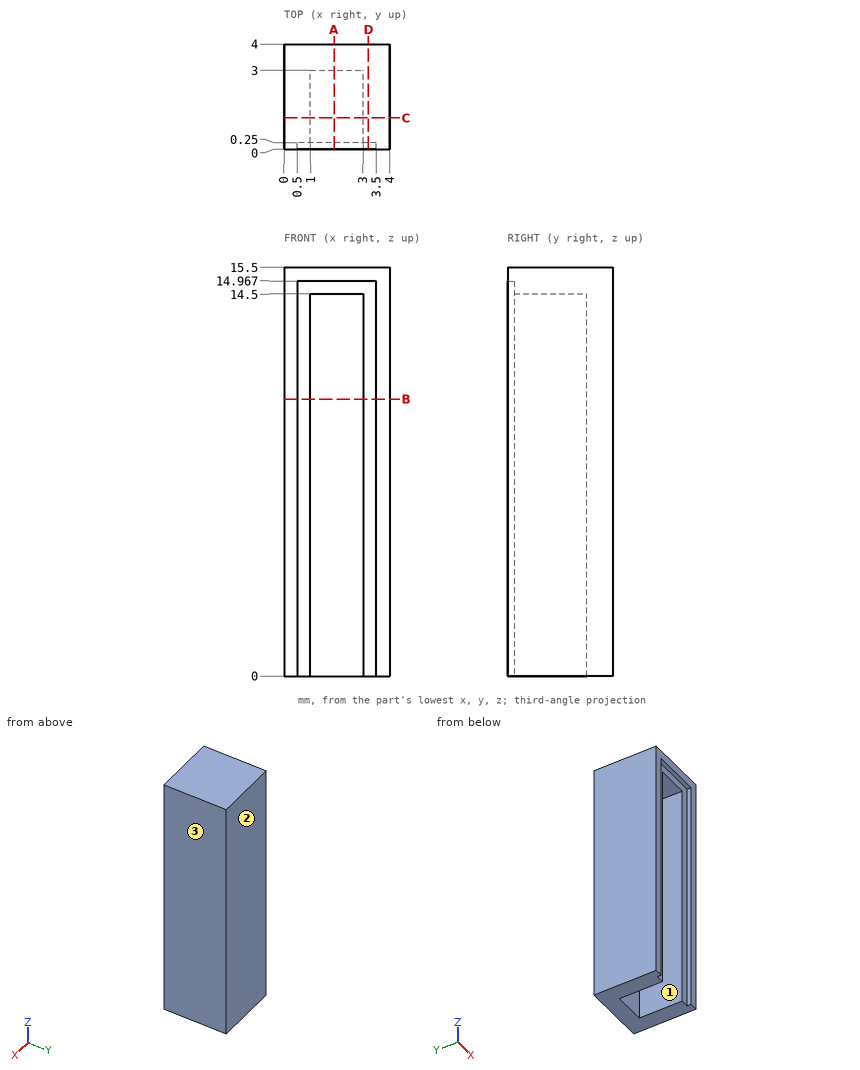
Could you check a few things on this drawing? It's one solid part, dimensions in mm from its lowest x, y, z. Round coordinates to 2 decimals unless told otherwise and drop trailing zeros. Order: outer loops, then holes, each group sorted by start corner. A loop starts at its lowest first (then second) coordinate and runs counter-clockwise, first axis right, second up. Notation, with made-up numbers: (-34.5, 40) -> (19.5, 40) arc R34 ccw to (19.5, 70) -> close; hole circle Ø1 at (76.25, -22.75). An arc over 180 degrees is marked (long way). One line per question, with ' | ' between items.
Q1. We'd pull the mould along X, two halves only. Please class the marked faces 1, 2 and 3: released by +X, released by -X, zero draft, split by the parting line, or undercut.
Computed values:
face 1: undercut | face 2: zero draft | face 3: released by +X
Q2. If I drill on line 1 (X direction, y = 1.9, z = 10.25); line 2 (Y direction, x = 1.65, z = 7); line 3 (Z direction, x = 1.9, y = 2.3), over which ranges is the centre line in solid material (lowest first)? Write a range as from..to.
Computed values:
line 1: 0..1, 3..4 | line 2: 3..4 | line 3: 14.5..15.5
Q3. I'm going to push flat-ended pins straight in: pin 1 (0.6 mm diameter, centred on x = 1.5, z = 9, fed in from -Y); pin 2 (1.5 mm diameter, centred on x = 2.5, z = 11, fed in from -Y). Where does each tip first touch, or does it pass through?
Computed values:
pin 1: y = 3 | pin 2: y = 0.25
Q4. If we section it at D-D on x = 3.2: Write out the boundary of the cut face in (y, z).
Computed values:
outline: (0, 14.97) -> (0.25, 14.97) -> (0.25, 0) -> (4, 0) -> (4, 15.5) -> (0, 15.5) -> close
Q5. If we section it at B-B on z = 10.5: Write out the boundary of the cut face in (x, y).
Computed values:
outline: (0, 0) -> (0.5, 0) -> (0.5, 0.25) -> (1, 0.25) -> (1, 3) -> (3, 3) -> (3, 0.25) -> (3.5, 0.25) -> (3.5, 0) -> (4, 0) -> (4, 4) -> (0, 4) -> close
Q6. If we section it at C-C on y = 1.2: Write out the boundary of the cut face in (x, z).
Computed values:
outline: (0, 0) -> (1, 0) -> (1, 14.5) -> (3, 14.5) -> (3, 0) -> (4, 0) -> (4, 15.5) -> (0, 15.5) -> close
Q7. If we section it at A-A on x = 1.9: Write out the boundary of the cut face in (y, z), plus the area to 3 significant figures.
Computed values:
outline: (0, 14.97) -> (0.25, 14.97) -> (0.25, 14.5) -> (3, 14.5) -> (3, 0) -> (4, 0) -> (4, 15.5) -> (0, 15.5) -> close | area: 18.4 mm²
